Input: part model. Units: mm. Frame: model coordinates. A direction names the side the tool comes from. Give positions to 0.01 mm unless a question says otherwise; leave off trailing zeros. Loops run counter-clockwise (first coordinate to the right, second up) from the corner with the lowest first, then second, coordinate; pieces in that order, holes last.
from build123d import *

# Parameters (mm, degrees)
SKETCH1_W           = 19.997483178
SKETCH1_H           = 15
SKETCH1_R           = 1.25
BOSS_EXTRUDE1_DEPTH = 4
SKETCH2_R           = 2.05
CUT_EXTRUDE1_DEPTH  = 2
FILLET1_R           = 1


with BuildPart() as part:
    # Sketch1 → Boss-Extrude1 (new body)
    with BuildSketch(Plane.XY):
        with Locations((0, -0.854350343)):
            Rectangle(SKETCH1_W, SKETCH1_H)
        with Locations((-4.851258411, -1.24229421)):
            Circle(SKETCH1_R, mode=Mode.SUBTRACT)
        with Locations((4.748741589, -1.24229421)):
            Circle(SKETCH1_R, mode=Mode.SUBTRACT)
    extrude(amount=BOSS_EXTRUDE1_DEPTH)

    # Sketch2 → Cut-Extrude1 (cut)
    with BuildSketch(Plane.XY.offset(4)):
        with Locations((-4.851258411, -1.24229421)):
            Circle(SKETCH2_R)
        with Locations((4.748741589, -1.24229421)):
            Circle(SKETCH2_R)
    extrude(amount=-CUT_EXTRUDE1_DEPTH, mode=Mode.SUBTRACT)

    # Fillet1
    fillet1_edges = [part.edges().sort_by_distance(p)[0] for p in [
        (9.998741589, -8.354350343, 2),
        (-9.998741589, -8.354350343, 2),
        (-9.998741589, 6.645649657, 2),
        (9.998741589, 6.645649657, 2),
    ]]
    fillet(fillet1_edges, radius=FILLET1_R)


solid = part.part
(1) Cut plane C-C (y = 0.5). Return the cut outline in (x, z), and give its area (3 significant figures).
Values follow:
outline: (-10, 0) - (10, 0) - (10, 4) - (5.83, 4) - (5.83, 2) - (3.67, 2) - (3.67, 4) - (-3.77, 4) - (-3.77, 2) - (-5.93, 2) - (-5.93, 4) - (-10, 4) - close
area: 71.3 mm2
(2) Cut plane A-A (x = -5). Return the cut outline in (y, z), and give its area (3 significant figures).
Values follow:
outline: (-8.35, 0) - (-2.48, 0) - (-2.48, 2) - (-3.29, 2) - (-3.29, 4) - (-8.35, 4) - close; (0, 0) - (6.65, 0) - (6.65, 4) - (0.8, 4) - (0.8, 2) - (0, 2) - close
area: 46.9 mm2
(3) Cut plane D-D (z = 3.65). Return the cut outline in (x, y).
Values follow:
outline: (-10, -7.35) arc R1 ccw to (-9, -8.35) - (9, -8.35) arc R1 ccw to (10, -7.35) - (10, 5.65) arc R1 ccw to (9, 6.65) - (-9, 6.65) arc R1 ccw to (-10, 5.65) - close; hole circle Ø4.1 at (-4.85, -1.24); hole circle Ø4.1 at (4.75, -1.24)
(4) Pin query (flat end, axial travel): pin 1 Ø1.2 at (x, y) = (-4, -2) entering from +Z. Return the tip coordinate at first contact, or that it passes through.
Values follow:
pin 1: stops at z = 2
(5) Ray query, probe 1 along X at (y, z) = (-0.75, 2.4); probe 2 along X at (y, z) = (-1, 3.2); probe 3 along Y at (x, z) = (4.75, 1.25). Return the intervals inside material, ascending.
Values follow:
probe 1: x = -10 to -6.84, -2.86 to 2.76, 6.74 to 10
probe 2: x = -10 to -6.89, -2.82 to 2.71, 6.78 to 10
probe 3: y = -8.35 to -2.49, 0.01 to 6.65
(6) Cut plane B-B (z = 0.9). Return the cut outline in (x, y).
Values follow:
outline: (-10, -7.35) arc R1 ccw to (-9, -8.35) - (9, -8.35) arc R1 ccw to (10, -7.35) - (10, 5.65) arc R1 ccw to (9, 6.65) - (-9, 6.65) arc R1 ccw to (-10, 5.65) - close; hole circle Ø2.5 at (-4.85, -1.24); hole circle Ø2.5 at (4.75, -1.24)
(7) Reachability of faces 1 (the cylindrical face through (-6.1, -1.2, 1)), 2 (the cylindrical face through (6.64, -2.03, 3.01)) from +Z, -Z, +X, -X, +Y, -Y: full face, straight path, thin tool, end or side. Return the list, or none.
Values follow:
face 1: +Z, -Z
face 2: +Z
(8) Mould query, pull axis Y, two halves, no side actions, for faces 3 (the flat face through (0, 6.646, 2)), 4 (the flat face through (-9.999, -1, 2)), 5 (the flat face through (-4, 0, 2)), 6 (the cylindrical face through (-9.714, -8.054, 2.028)). Classes: +Y half, -Y half, draft (parallel to the pull), parting line (faces both ways), or undercut.
Values follow:
face 3: +Y half
face 4: draft
face 5: undercut
face 6: -Y half
